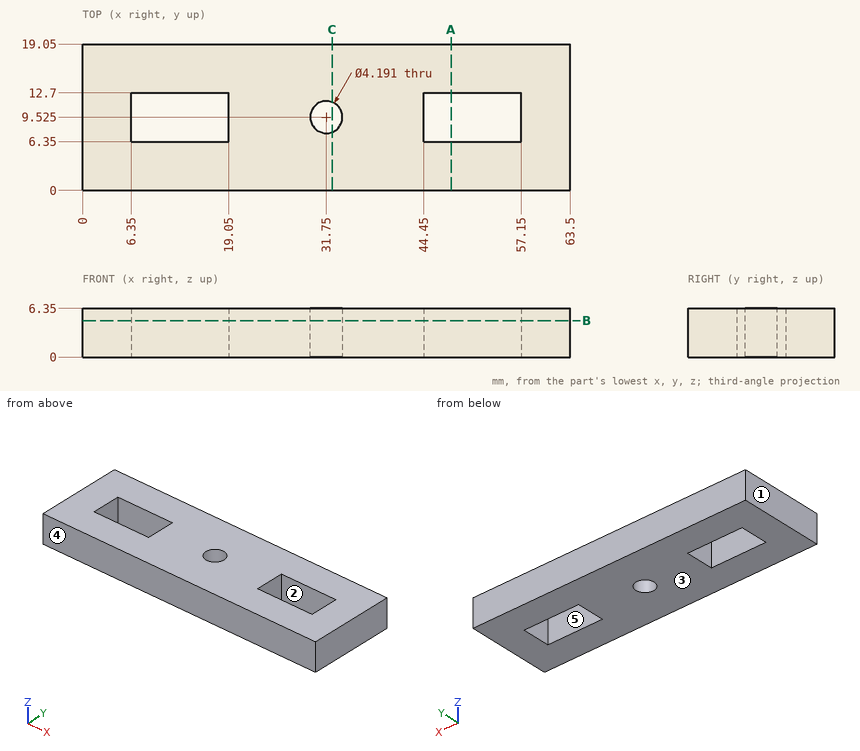
For this review, use the dimensioned drawing (mm, ordinates from the lowest corner) and the shaded views. A direction names the side the tool comes from. Give positions to 0.01 mm unless a question says otherwise; leave off trailing zeros. Write each loop counter-clockwise with the first axis right and the second up, starting at its lowest first coordinate (ties: lowest second). Pieces come first, ordered by that corner, then holes. Notation, with made-up numbers: M 83,-28.75 L 142,-28.75 A13 ccw 142,-5.75 Z; hole C 55,78.25 d6. An arc over 180 degrees is marked long. Write item = value, one per line. Start each with the question number.
Q1. Clearance check with flat-ended pins moving along their axes: pin 1 (3 mm diameter, centred on y = 8.5, z = 4.5, fed in from -X); pin 2 (3.5 mm diameter, centred on x = 31.75, y = 9.525, fed in from +Z). State where each tip first meets the part, or that it passes through.
Q2. Mouldability with a two-part tool opening along X and no side actions: class the marked faces 1, 2 and 3 as released by +X, released by -X, zero draft, split by the parting line, or undercut.
Q3. For line 1 (X direction, y = 12.5, z = 3); line 2 (X direction, y = 8.5, z = 2.25); line 3 (Y direction, x = 9.5, z = 1.25), list the stretches that pass through material, from the lowest coordinate up.
Q4. We need section B-B (z = 4.75). Give the number of separate pieces and of enclosed holes in the cut face, plus the area to 3 significant figures.
Q5. We need section C-C (x = 32.5). State the section outline as (y, z) points.
Q6. We need section A-A (x = 48). State the section outline as (y, z) points.
Q7. Machinability: for the marked faces 4 and 5, which of the approach directions +Z, -Z, +X, -X, +Y, -Y give a long, thin tool a straight path to every point of the face, cutting with its end or side? Answer none if there is none.
Result set:
q1.pin_1 = 0
q1.pin_2 = through
q2.face_1 = released by -X
q2.face_2 = undercut
q2.face_3 = zero draft
q3.line_1 = 0 to 6.35, 19.05 to 44.45, 57.15 to 63.5
q3.line_2 = 0 to 6.35, 19.05 to 29.92, 33.58 to 44.45, 57.15 to 63.5
q3.line_3 = 0 to 6.35, 12.7 to 19.05
q4.separate_pieces = 1
q4.enclosed_holes = 3
q4.area = 1,030 mm2
q5.outline = M 0,0 L 7.57,0 L 7.57,6.35 L 0,6.35 Z; M 11.48,0 L 19.05,0 L 19.05,6.35 L 11.48,6.35 Z
q6.outline = M 0,0 L 6.35,0 L 6.35,6.35 L 0,6.35 Z; M 12.7,0 L 19.05,0 L 19.05,6.35 L 12.7,6.35 Z
q7.face_4 = +Z, -Z, +X, -X, -Y
q7.face_5 = +Z, -Z
